```python
from build123d import *

# Parameters (mm, degrees)
ESBO_O1_R                = 48
RESSALTO_EXTRUS_O1_DEPTH = 5
ESBO_O2_R                = 5
RESSALTO_EXTRUS_O2_DEPTH = 15
ESBO_O3_R                = 10
RESSALTO_EXTRUS_O4_DEPTH = 10


with BuildPart() as part:
    # Esboço1 → Ressalto-extrusão1 (new body)
    with BuildSketch(Plane.XY):
        Circle(ESBO_O1_R)
    extrude(amount=RESSALTO_EXTRUS_O1_DEPTH)

    # Esboço2 → Ressalto-extrusão2 (add)
    with BuildSketch(Plane.XY):
        with Locations((0, 40)):
            Circle(ESBO_O2_R)
    extrude(amount=RESSALTO_EXTRUS_O2_DEPTH)

    # Esboço3 → Ressalto-extrusão4 (add)
    with BuildSketch(Plane(origin=(0, 0, 0), x_dir=(-1, 0, 0), z_dir=(0, 0, -1))):
        Circle(ESBO_O3_R)
    extrude(amount=RESSALTO_EXTRUS_O4_DEPTH)


solid = part.part
```
Geometry check sheet. Reference: the model listing, model coordinates, mm. A direction names the side the tool comes from. Coordinates: 2 decimals unless noted, no trailing zeros. Order: outer loops, then holes, each group sorted by start corner. A loop starts at its lowest first (then second) coordinate and runs counter-clockwise, first axis right, second up. Notation, with made-up numbers: M 44.5,27 L 49.5,27 A28 cw 49.5,62 Z; hole C 79.5,57 d9. An arc over 180 degrees is marked long. One line per question, with ' | ' between items. Start each with the question number.
Item 1: Material ranges on L1, parallel to Z at x = -35.5, y = 1; L2, parallel to Z at x = -2.5, y = -8; L3, parallel to Y at x = -13, z = 2.5, recorded low to high. Write a range as [from, to].
Item 2: Cross-section at B-B on y = 0. Enter the section's corners in (x, z).
Item 3: Gauge pin test, flat ends, axial feed: pin 1 (2 mm diameter, centred on x = 26, y = -2.5, fed in from +Z); pin 2 (1 mm diameter, centred on x = -37, z = 2, fed in from -Y); pin 3 (1 mm diameter, centred on x = -15, y = -34, fed in from -Z). Record the tip position at first contact, or that the pin passes through.
Item 4: Cross-section at A-A on x = 0. Enter the section's corners in (y, z), then the cut area to 3 significant figures.
Item 5: Cross-section at C-C on z = -3. Enter the section's corners in (x, y).
Item 6: Cross-section at D-D on z = 9. Enter the section's corners in (x, y), then the cut area to 3 significant figures.
Item 7: Set-up check for faces 1 (the cylindrical face through (-0.651, 44.957, 9.93)), 2 (the flat face through (-1, 11, 0)), 3 (the flat face through (0, 0, -10)): record each of +Z, -Z, +X, -X, +Y, -Y from which the full face is reachable in a straight line by a thin tool's end or side.
Findings:
1) L1: z = [0, 5] | L2: z = [-10, 5] | L3: y = [-46.21, 46.21]
2) outline: M -48,0 L -10,0 L -10,-10 L 10,-10 L 10,0 L 48,0 L 48,5 L -48,5 Z
3) pin 1: stops at z = 5 | pin 2: stops at y = -31.17 | pin 3: stops at z = 0
4) outline: M -48,0 L -10,0 L -10,-10 L 10,-10 L 10,0 L 48,0 L 48,5 L 45,5 L 45,15 L 35,15 L 35,5 L -48,5 Z | area: 780 mm²
5) outline: C 0,0 d20
6) outline: C 0,40 d10 | area: 78.5 mm²
7) face 1: +Z | face 2: -Z | face 3: -Z, +X, -X, +Y, -Y
